Geometry check sheet. Reference: the model listing, model coordinates, mm. Round coordinates to 2 decimals unless told otherwise and drop trailing zeros. Loops run counter-clockwise (first coordinate to the right, second up) from the corner with the lowest first, then second, coordinate; pieces in that order, holes last. Notation, with made-up numbers: (-4, 68) -> (28, 68) arc R21 ccw to (28, 105) -> close; hole circle Ø7 at (-31.75, 58). An arc over 180 degrees is marked (long way). Use one line per item in the form item = value.
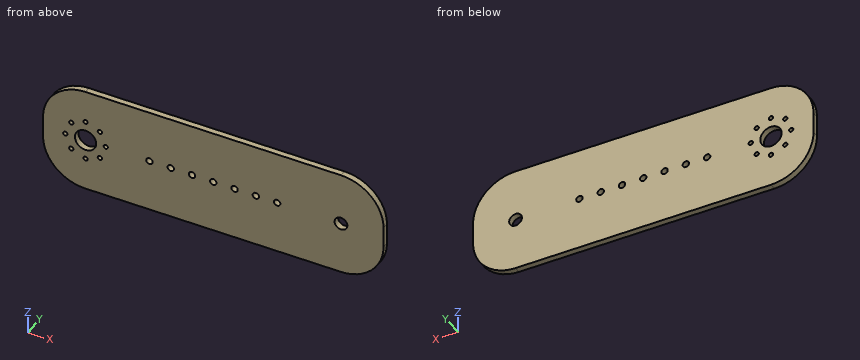
from build123d import *

# Parameters (mm, degrees)
SKETCH1_W           = 160
SKETCH1_H           = 50
BOSS_EXTRUDE1_DEPTH = 3
FILLET1_R           = 20
SKETCH2_R           = 5
CUT_EXTRUDE1_DEPTH  = 4
SKETCH3_R           = 1
CUT_EXTRUDE2_DEPTH  = 4
CIRPATTERN1_COUNT   = 8
SKETCH4_R           = 3
CUT_EXTRUDE3_DEPTH  = 4
SKETCH5_R           = 1.5
CUT_EXTRUDE4_DEPTH  = 4
LPATTERN1_COUNT     = 4
LPATTERN1_PITCH     = 10
LPATTERN1_COL_COUNT = 4
LPATTERN1_COL_PITCH = 10


with BuildPart() as part:
    # Sketch1 → Boss-Extrude1 (new body)
    with BuildSketch(Plane(origin=(0, 0, 0), x_dir=(1, 0, 0), z_dir=(0, 1, 0))):
        Rectangle(SKETCH1_W, SKETCH1_H)
    extrude(amount=BOSS_EXTRUDE1_DEPTH)

    # Fillet1
    fillet1_edges = [part.edges().sort_by_distance(p)[0] for p in [
        (80, 1.5, 25),
        (-80, 1.5, 25),
        (-80, 1.5, -25),
        (80, 1.5, -25),
    ]]
    fillet(fillet1_edges, radius=FILLET1_R)

    # Sketch2 → Cut-Extrude1 (cut, through all)
    with BuildSketch(Plane(origin=(0, 3, 0), x_dir=(1, 0, 0), z_dir=(0, 1, 0))):
        with Locations((-60, 0)):
            Circle(SKETCH2_R)
    extrude(amount=-CUT_EXTRUDE1_DEPTH, mode=Mode.SUBTRACT)

    # Sketch3 → Cut-Extrude2 (cut, through all)
    with BuildSketch(Plane(origin=(0, 3, 0), x_dir=(1, 0, 0), z_dir=(0, 1, 0))):
        with Locations((-50.5, 0)):
            Circle(SKETCH3_R)
    cut_extrude2 = extrude(amount=-CUT_EXTRUDE2_DEPTH, mode=Mode.SUBTRACT)

    # CirPattern1: Cut-Extrude2 ×8 about axis
    cirpattern1_axis = Axis((-60, 0, 0), (0, 1, 0))
    for i in range(1, CIRPATTERN1_COUNT):
        add(cut_extrude2.rotate(cirpattern1_axis, i * 360 / CIRPATTERN1_COUNT), mode=Mode.SUBTRACT)

    # Sketch4 → Cut-Extrude3 (cut, through all)
    with BuildSketch(Plane(origin=(0, 3, 0), x_dir=(1, 0, 0), z_dir=(0, 1, 0))):
        with Locations((60, 0)):
            Circle(SKETCH4_R)
    extrude(amount=-CUT_EXTRUDE3_DEPTH, mode=Mode.SUBTRACT)

    # Sketch5 → Cut-Extrude4 (cut, through all)
    with BuildSketch(Plane(origin=(0, 3, 0), x_dir=(1, 0, 0), z_dir=(0, 1, 0))):
        Circle(SKETCH5_R)
    cut_extrude4 = extrude(amount=-CUT_EXTRUDE4_DEPTH, mode=Mode.SUBTRACT)

    # LPattern1: Cut-Extrude4 ×4
    with Locations(*[(i * LPATTERN1_PITCH, 0, 0) for i in range(1, LPATTERN1_COUNT)]):
        add(cut_extrude4, mode=Mode.SUBTRACT)

    # LPattern1 col: Cut-Extrude4 ×4
    with Locations(*[(-i * LPATTERN1_COL_PITCH, 0, 0) for i in range(1, LPATTERN1_COL_COUNT)]):
        add(cut_extrude4, mode=Mode.SUBTRACT)


solid = part.part
1. Gauge pin test, flat ends, axial feed: pin 1 (10 mm diameter, centred on x = -62.5, z = 18.5, fed in from -Y); pin 2 (2.5 mm diameter, centred on x = -30, z = 0, fed in from -Y). Record the tip position at first contact, or that the pin passes through.
Return value:
pin_1 = 0
pin_2 = through
2. Material ranges on line 1 along Z through (x, y) = (-30, 1.75); line 2 along Z through (x, y) = (58.5, 1.8); line 3 along X through (y, z) = (2.6, -4), recorded low to high.
Return value:
line_1 = -25 to -1.5, 1.5 to 25
line_2 = -25 to -2.6, 2.6 to 25
line_3 = -80 to -63, -57 to 80
3. Section check C-C (x = 68). Record the boundary of the cut face in (y, z).
Return value:
outline = (0, -23.33) -> (3, -23.33) -> (3, 23.33) -> (0, 23.33) -> close
4. Section check B-B (y = 2.1). Count the separate pieces of the cut face and the enclosed holes in it, then the cut area to 3 significant figures.
Return value:
separate_pieces = 1
enclosed_holes = 17
area = 7,480 mm2
5. Section check A-A (x = 20). Record the boundary of the cut face in (y, z).
Return value:
outline = (0, -25) -> (3, -25) -> (3, -1.5) -> (0, -1.5) -> close; (0, 1.5) -> (3, 1.5) -> (3, 25) -> (0, 25) -> close
